from build123d import *

# Parameters (mm, degrees)
F0_R     = 33
F1_DEPTH = 30
F2_T     = -2
F3_DEPTH = 109
F4_W     = 28
F4_H     = 28
F5_DEPTH = 12.5


# Not quite as in the source:
# - an extrude ends at something that could not be found from the text; its depth is read off the source's solid


with BuildPart() as f1:
    # F0 (on Top) → F1 (new body)
    with BuildSketch(Plane.XY):
        Circle(F0_R)
    extrude(amount=F1_DEPTH)

    # F2
    f2_openings = [f1.faces().sort_by_distance(p)[0] for p in [
        (0, 0, 30),
    ]]
    offset(amount=F2_T, openings=f2_openings)

    # F0 (on Top) → F3 (cut, through all)
    with BuildSketch(Plane.XY):
        Circle(F0_R)
    extrude(amount=-F3_DEPTH, mode=Mode.SUBTRACT)

    # F4 (on face) → F5 (cut, symmetric)
    with BuildSketch(Plane.XY):
        Rectangle(F4_W, F4_H)
    extrude(amount=F5_DEPTH, both=True, mode=Mode.SUBTRACT)


solid = f1.part
Model file for the job. Use its own axes, mm. A direction names the side the tool comes from. Give positions to 0.01 mm unless a question says otherwise; leave off trailing zeros. Order: outer loops, then holes, each group sorted by start corner. A loop starts at its lowest first (then second) coordinate and runs counter-clockwise, first axis right, second up. Notation, with made-up numbers: M 15.25,5.5 L 19.25,5.5 A18 cw 19.25,33.5 Z; hole C 39.25,-23 d10. An arc over 180 degrees is marked long. Write item = value, one per line.
Q1. Two-plate mould, pull along Y, no slides. Class faces 3 (the cylindrical face through (30.5, -12.6, 14.8)), 4 (the flat face through (-0.5, -14.2, 0)), 5 (the flat face through (0, 14, 1)): pulls with the +Y half, pulls with the -Y half, needs draft (parallel to the pull), parting line crosses it, or undercut.
Derived:
face_3 = parting line crosses it
face_4 = needs draft
face_5 = undercut
Q2. Flat gauge pins, fed straight in: pin 1 (1.6 mm diameter, centred on y = 1.5, z = 1.5, fed in from -X); pin 2 (1 mm diameter, centred on x = 3.5, z = 26, fed in from -Y); pin 3 (3 mm diameter, centred on y = 19.5, z = 17, fed in from -X). Where does each tip first touch, or does it go through?
Derived:
pin_1 = -32.99
pin_2 = -32.86
pin_3 = -27.66
Q3. Cut at D-D, the plane y = -28. List the corners of the cut face in (x, z), then the cut area to 3 significant figures.
Derived:
outline = M -17.46,0 L 17.46,0 L 17.46,30 L 13.3,30 L 13.3,2 L -13.3,2 L -13.3,30 L -17.46,30 Z
area = 303 mm2
Q4. Cut at A-A, the plane x = 0. List the corners of the cut face in (y, z), then the cut area to 3 significant figures.
Derived:
outline = M -33,0 L -14,0 L -14,2 L -31,2 L -31,30 L -33,30 Z; M 14,0 L 33,0 L 33,30 L 31,30 L 31,2 L 14,2 Z
area = 188 mm2
Q5. Drill centre lines: line 1 (Y direction, x = 0, z = 11); line 2 (Z direction, x = -2, y = -20); line 3 (X direction, y = -13.5, z = 13.75). Where is each one in solid material? Low to high. Write a range as [from, to].
Derived:
line_1 = [-33, -31], [31, 33]
line_2 = [0, 2]
line_3 = [-30.11, -27.91], [27.91, 30.11]
Q6. Cut at C-C, the plane z = 21.75. List the corners of the cut face in (x, y), then the cut area to 3 significant figures.
Derived:
outline = C 0,0 d66; hole C 0,0 d62
area = 402 mm2
Q7. Tool access for faces 1 (the cylindrical face through (-4.036, 30.736, 15.804)), 2 (the flat face through (-14, 0, 1)): list every direction of +Z, -Z, +X, -X, +Y, -Y with a clear straight run to the whole face (end or side of a thin tool).
Derived:
face_1 = +Z
face_2 = +Z, -Z
